Can you work these out from the drawing? Everything is in mm from the part's minimum corner. A direction names the side the tool comes from. Give positions to 0.01 mm unless a question says otherwise; leave off trailing zeros. Loops run counter-clockwise (first coordinate to the right, second up) from the corner with the lowest first, then second, coordinate; pieces in that order, holes last. Notation, with made-up numbers: (34, 20.25) -> (71, 20.25) arc R10 cw to (71, 33.25) -> close; hole circle Ø10 at (83.5, -29.5). An arc over 180 degrees is marked (long way). Return JSON: item names as keys, results as strings. Group by question number.
Q1. Suppose I cut it at D-D, the plane y = 61. Please give me the cut outline in (x, z).
Q2. Which directions (+Z, -Z, +X, -X, +Y, -Y) give clear straight access to the entire face, cutting with the end or side of a thin tool? Please do the marked faces 4 and 5.
Q3. Suppose I cut it at C-C, the plane x = 217.5. Please give me the cut outline in (y, z), and give its area (3 significant figures).
Q4. Will these pins go through, and if not, where does the flat tip stop? pin 1 (12 mm diameter, centred on x = 200, z = 52, fed in from -Y); pin 2 (1.5 mm diameter, centred on x = 320, z = 80.5, fed in from +Y); pin 3 (1 mm diameter, centred on x = 325.5, z = 50, fed in from -Y).
Q5. Thinking about a two-plate mould opening in X: for the marked faces 1, 2 and 3, which applies, pulls with the +X half, pulls with the -X half, needs draft (parallel to the pull), parting line crosses it, or undercut?
Q6. Suppose I cut it at B-B, the plane z = 114. Please give me the cut outline in (x, y).
Q7. I need wall thicknesses on line 1 along Y through (x, z) = (278, 80); line 2 along X through (y, z) = (10, 14.5); line 3 along X through (y, z) = (30, 47). Which ranges of each line are inside material? Lowest first, please. Write a range as [from, to].
Q8. Suppose I cut it at A-A, the plane y = 18. Please give me the cut outline in (x, z), and give its area (3 significant figures).
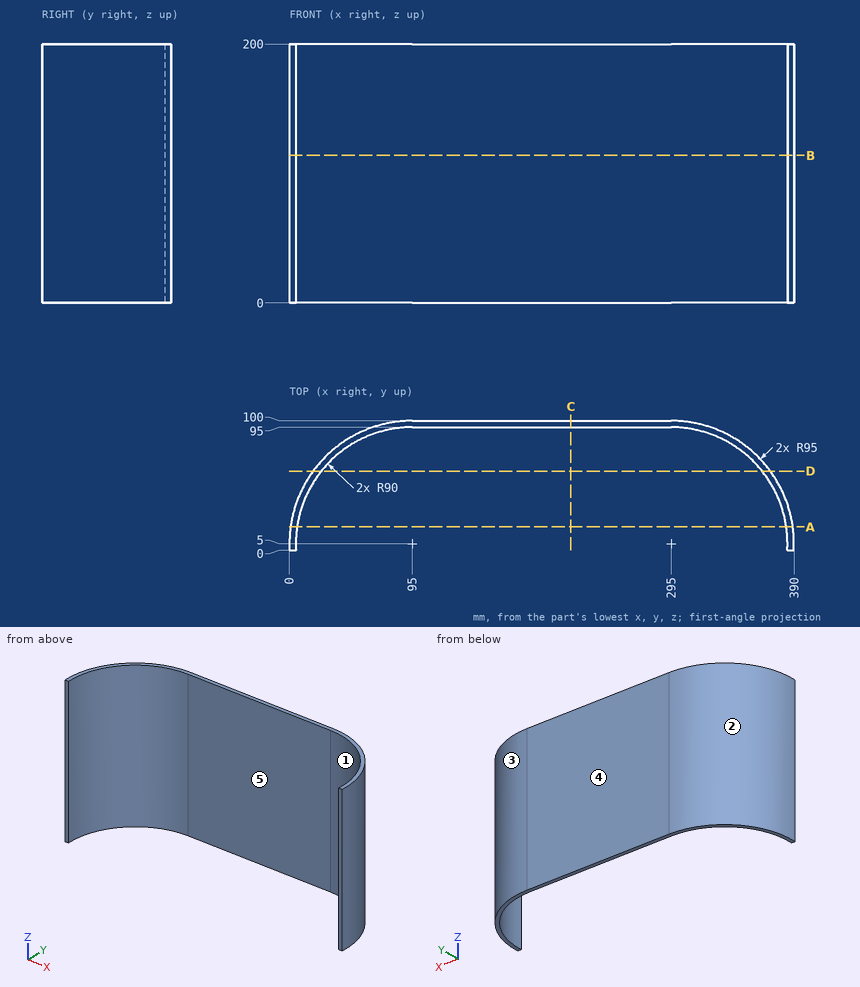
Ans:
{
 "1": {"outline": "(18.26, 0) -> (24.54, 0) -> (24.54, 200) -> (18.26, 200) -> close; (365.46, 0) -> (371.74, 0) -> (371.74, 200) -> (365.46, 200) -> close"},
 "2": {"face 4": "+Z, -Z, +X, -X, +Y", "face 5": "+Z, -Z, -Y"},
 "3": {"outline": "(95, 0) -> (100, 0) -> (100, 200) -> (95, 200) -> close", "area": "1,000 mm^2"},
 "4": {"pin 1": "stops at y = 95", "pin 2": "stops at y = 96.85", "pin 3": "stops at y = 89.49"},
 "5": {"face 1": "undercut", "face 2": "pulls with the -X half", "face 3": "pulls with the +X half"},
 "6": {"outline": "(0.13, 0) -> (5.14, 0) arc R90 cw to (95, 95) -> (295, 95) arc R90 cw to (384.86, 0) -> (389.87, 0) arc R95 ccw to (295, 100) -> (95, 100) arc R95 ccw to start"},
 "7": {"line 1": "y = [95, 100]", "line 2": "x = [0.13, 5.14], [384.86, 389.87]", "line 3": "x = [3.35, 8.54], [381.46, 386.65]"},
 "8": {"outline": "(0.89, 0) -> (5.94, 0) -> (5.94, 200) -> (0.89, 200) -> close; (384.06, 0) -> (389.11, 0) -> (389.11, 200) -> (384.06, 200) -> close", "area": "2,020 mm^2"}
}
